from build123d import *

# Parameters (mm, degrees)
SALIENTE_EXTRUIR1_DEPTH = 25
REDONDEO1_R             = 20


with BuildPart() as part:
    # Croquis1 → Saliente-Extruir1 (new, symmetric)
    with BuildSketch(Plane.XY):
        Polygon((0, 8), (0, 0), (-90, 0), (-90, 74.370702608), (-24.226182617, 105.04153736), (-20, 95.978459489), (-80, 68), (-80, 8), align=None)
    extrude(amount=SALIENTE_EXTRUIR1_DEPTH, both=True)

    # Redondeo1
    redondeo1_edges = [part.edges().sort_by_distance(p)[0] for p in [
        (-90, 74.370702608, 0),
        (-80, 68, 0),
    ]]
    fillet(redondeo1_edges, radius=REDONDEO1_R)


solid = part.part
Verification items for the finished model (mm, model axes). A direction names the side the tool comes from. Coordinates: 2 decimals unless noted, no trailing zeros. Write each loop counter-clockwise with the first axis right and the second up, starting at its lowest first coordinate (ties: lowest second). Pieces come first, ordered by that corner, then holes. Notation, with made-up numbers: (43.25, 21.25) -> (49.25, 21.25) arc R17 ccw to (49.25, 45.25) -> close; hole circle Ø3 at (-30, 49). An arc over 180 degrees is marked (long way). One line per item, written item: value. Start each with the question number.
Q1. Cross-section at A-A on x = -22. Enter the section's corners in (y, z).
Q2. Go/stop test with flat-tipped pins: P1, Ø5, axis at y = 75.5, z = -17.5, coming from the -X side; P2, Ø6, axis at y = 91.5, z = -16, coming from the +X side; P3, Ø1, axis at y = 13.5, z = -4, coming from the +X side. Record where each tip stops, or that it passes through.
Q3. Access from +Z, -Z, +X, -X, +Y, -Y to the whole of each face (thin tool, end or side, straight path). Record for faces 5 (the flat face through (-41, 8, 0)), 6 (the flat face through (-22.14, 100.57, 0.35)).
Q4. Cross-section at C-C on x = -6.5. Enter the section's corners in (y, z).
Q5. Mould release check, pull along Y, two halves, no side actions. Record for faces 1 (the cylindrical face through (-76.953, 65.87, 0.35)), 2 (the flat face through (-51.72, 92.22, 0.35)), 3 (the flat face through (-81, 45, 25)), 4 (the flat face through (-43.89, 84.84, 0.35)): pulls with the +Y half, pulls with the -Y half, needs draft (parallel to the pull), parting line crosses it, or undercut.
Q6. Thickness scan on L1, parallel to X at y = 47.5, z = 9.5; L2, parallel to Y at x = -63, z = 0; L3, parallel to Y at x = -12, z = -3. Record the ranges inside material, lowest first. Write a range as from..to.
Q7. Cross-section at B-B on z = -6.5. Enter the section's corners in (x, y), and give its area (3 significant figures).
Q8. Cross-section at D-D on y = 17. Enter the section's corners in (x, z).
Checked values:
1. outline: (0, -25) -> (8, -25) -> (8, 25) -> (0, 25) -> close; (95.05, -25) -> (100.27, -25) -> (100.27, 25) -> (95.05, 25) -> close
2. P1: stops at x = -86.45
2. P2: stops at x = -23.17
2. P3: stops at x = -80
3. face 5: +Z, -Z, +X
3. face 6: +Z, -Z, +X, +Y
4. outline: (0, -25) -> (8, -25) -> (8, 25) -> (0, 25) -> close
5. face 1: undercut
5. face 2: pulls with the +Y half
5. face 3: needs draft
5. face 4: undercut
6. L1: x = -90..-80
6. L2: y = 0..8, 75.93..86.96
6. L3: y = 0..8
7. outline: (-90, 0) -> (0, 0) -> (0, 8) -> (-80, 8) -> (-80, 55.26) arc R20 cw to (-68.45, 73.38) -> (-20, 95.98) -> (-24.23, 105.04) -> (-78.45, 79.76) arc R20 ccw to (-90, 61.63) -> close
7. area: 2,050 mm²
8. outline: (-90, -25) -> (-80, -25) -> (-80, 25) -> (-90, 25) -> close
